CAD build for the part. Positions are in the model's coordinates, mm. A direction names the side the tool comes from. Coordinates: 2 decimals unless noted, no trailing zeros. Loops run counter-clockwise (first coordinate to the right, second up) from the corner with the lowest first, then second, coordinate; pieces in that order, holes last. Notation, with made-up numbers: (-31, -7.5) - (-11, -7.5) arc R19 cw to (-11, -1.5) - close; hole circle Ø2 at (26, -31.5). An arc over 180 degrees is marked (long way). Put each result on its own line as item: value.
```python
from build123d import *
from build123d.topology import SkipClean

# Parameters (mm, degrees)
SKETCH1_R           = 254.5
SKETCH1_R_2         = 234.5
BOSS_EXTRUDE1_DEPTH = 5
BOSS_EXTRUDE2_DEPTH = 500
SKETCH3_W           = 27.805822748
SKETCH3_H           = 60
CUT_EXTRUDE1_DEPTH  = 500
SKETCH4_R           = 250.5
CUT_EXTRUDE2_DEPTH  = 500
BOSS_EXTRUDE3_DEPTH = 500
BOSS_EXTRUDE4_DEPTH = 5
SKETCH11_W          = 21.416490723
SKETCH11_H          = 190
CUT_EXTRUDE3_DEPTH  = 10
CUT_EXTRUDE4_DEPTH  = 10
FILLET1_R           = 5
SKETCH15_R          = 2.5
CUT_EXTRUDE5_DEPTH  = 10
BOSS_EXTRUDE5_DEPTH = 3
SKETCH18_R          = 2.5
CUT_EXTRUDE6_DEPTH  = 5
CUT_EXTRUDE7_DEPTH  = 7
FILLET2_R           = 5
SKETCH21_R          = 2.5
CUT_EXTRUDE8_DEPTH  = 10
SKETCH22_R          = 2.5
CUT_EXTRUDE9_DEPTH  = 14
SKETCH23_R          = 5
CUT_EXTRUDE10_DEPTH = 3
SKETCH24_W          = 28.197779234
SKETCH24_H          = 25
CUT_EXTRUDE11_DEPTH = 45
FILLET3_R           = 2


with BuildPart() as part:
    # Sketch1 → Boss-Extrude1 (new body)
    with BuildSketch(Plane(origin=(0, 0, 0), x_dir=(1, 0, 0), z_dir=(0, 1, 0))):
        with Locations(Location((0, 0, 0), (0, 0, 270))):
            Circle(SKETCH1_R)
        with Locations(Location((0, 0, 0), (0, 0, 270))):
            Circle(SKETCH1_R_2, mode=Mode.SUBTRACT)
    extrude(amount=BOSS_EXTRUDE1_DEPTH)

    # Sketch2 → Boss-Extrude2 (add)
    with SkipClean():  # the faces are left unmerged after this step: merging them gives an invalid solid
        with BuildSketch(Plane(origin=(0, 5, 0), x_dir=(1, 0, 0), z_dir=(0, 1, 0))):
            with BuildLine():
                Line((254.5, 0), (234.5, 0))
                ThreePointArc((234.5, 0), (225.296071541, 65.053286992), (198.406779118, 125))
                Line((198.406779118, 125), (221.687279743, 125))
                ThreePointArc((221.687279743, 125), (246.16017417, 64.617479467), (254.5, 0))
            make_face()
        boss_extrude2 = extrude(amount=BOSS_EXTRUDE2_DEPTH)

    # Mirror1: Boss-Extrude2 across plane
    with SkipClean():  # the faces are left unmerged after this step: merging them gives an invalid solid
        add(boss_extrude2.mirror(Plane(origin=(0, 505, 0), x_dir=(1, 0, 0), z_dir=(0, 0, 1))))

    # Sketch3 → Cut-Extrude1 (cut)
    with SkipClean():  # the faces are left unmerged after this step: merging them gives an invalid solid
        with BuildSketch(Plane(origin=(0, 5, 0), x_dir=(1, 0, 0), z_dir=(0, 1, 0))):
            with Locations((-240.597088626, 30)):
                Rectangle(SKETCH3_W, SKETCH3_H)
        cut_extrude1 = extrude(amount=-CUT_EXTRUDE1_DEPTH, mode=Mode.SUBTRACT)

    # Mirror2: Cut-Extrude1 across plane
    with SkipClean():  # the faces are left unmerged after this step: merging them gives an invalid solid
        add(cut_extrude1.mirror(Plane.XY), mode=Mode.SUBTRACT)

    # Sketch4 → Cut-Extrude2 (cut)
    with SkipClean():  # the faces are left unmerged after this step: merging them gives an invalid solid
        with BuildSketch(Plane(origin=(0, 505, 0), x_dir=(1, 0, 0), z_dir=(0, 1, 0))):
            Circle(SKETCH4_R)
        extrude(amount=-CUT_EXTRUDE2_DEPTH, mode=Mode.SUBTRACT)

    # Sketch8 → Boss-Extrude3 (add)
    with SkipClean():  # the faces are left unmerged after this step: merging them gives an invalid solid
        with BuildSketch(Plane(origin=(0, 5, 0), x_dir=(1, 0, 0), z_dir=(0, 1, 0))):
            Polygon((217.083509277, 125), (168.583509277, 125), (168.583509277, 120), (220.045796136, 120), (220.045796136, 125), align=None)
        boss_extrude3 = extrude(amount=BOSS_EXTRUDE3_DEPTH)

    # Mirror3: Boss-Extrude3 across plane
    with SkipClean():  # the faces are left unmerged after this step: merging them gives an invalid solid
        add(boss_extrude3.mirror(Plane.XY))

    # Sketch10 → Boss-Extrude4 (add)
    with SkipClean():  # the faces are left unmerged after this step: merging them gives an invalid solid
        with BuildSketch(Plane.XZ):
            with BuildLine():
                Line((198.406779118, 125), (168.583509277, 125))
                Line((168.583509277, 125), (168.583509277, -125))
                Line((168.583509277, -125), (198.406779118, -125))
                ThreePointArc((198.406779118, -125), (234.5, 0), (198.406779118, 125))
            make_face()
        extrude(amount=-BOSS_EXTRUDE4_DEPTH)

    # Sketch11 → Cut-Extrude3 (cut)
    with SkipClean():  # the faces are left unmerged after this step: merging them gives an invalid solid
        with BuildSketch(Plane(origin=(0, 5, 0), x_dir=(1, 0, 0), z_dir=(0, 1, 0))):
            with Locations((179.291754639, -1.5)):
                Rectangle(SKETCH11_W, SKETCH11_H)
        extrude(amount=-CUT_EXTRUDE3_DEPTH, mode=Mode.SUBTRACT)

    # Sketch12 → Cut-Extrude4 (cut)
    with SkipClean():  # the faces are left unmerged after this step: merging them gives an invalid solid
        with BuildSketch(Plane(origin=(0, 5, 0), x_dir=(1, 0, 0), z_dir=(0, 1, 0))):
            with BuildLine():
                Line((213, 93.5), (190, 93.5))
                Line((190, 93.5), (190, 75))
                Line((190, 75), (213, 75))
                ThreePointArc((213, 75), (216.535533906, 76.464466094), (218, 80))
                Line((218, 80), (218, 88.5))
                ThreePointArc((218, 88.5), (216.535533906, 92.035533906), (213, 93.5))
            make_face()
            with BuildLine():
                Line((185, 120), (168.583509277, 120))
                Line((168.583509277, 120), (168.583509277, 93.5))
                Line((168.583509277, 93.5), (190, 93.5))
                Line((190, 93.5), (190, 115))
                ThreePointArc((190, 115), (188.535533906, 118.535533906), (185, 120))
            make_face()
            with BuildLine():
                ThreePointArc((213, -93.5), (216.535533906, -92.035533906), (218, -88.5))
                Line((218, -88.5), (218, -80))
                ThreePointArc((218, -80), (216.535533906, -76.464466094), (213, -75))
                Line((213, -75), (190, -75))
                Line((190, -75), (190, -93.5))
                Line((190, -93.5), (213, -93.5))
            make_face()
            with BuildLine():
                Line((190, -115), (190, -93.5))
                Line((190, -93.5), (168.583509277, -93.5))
                Line((168.583509277, -93.5), (168.583509277, -120))
                Line((168.583509277, -120), (185, -120))
                ThreePointArc((185, -120), (188.535533906, -118.535533906), (190, -115))
            make_face()
        extrude(amount=-CUT_EXTRUDE4_DEPTH, mode=Mode.SUBTRACT)

    # Fillet1
    fillet1_edges = [part.edges().sort_by_distance(p)[0] for p in [
        (190, 2.5, 75),
        (190, 2.5, 93.5),
        (190, 2.5, -93.5),
        (190, 2.5, -75),
    ]]
    fillet(fillet1_edges, radius=FILLET1_R)

    # Sketch15 → Cut-Extrude5 (cut)
    with BuildSketch(Plane(origin=(0, 5, 0), x_dir=(1, 0, 0), z_dir=(0, 1, 0))):
        with Locations(Location((242.5, 0, 0), (0, 0, 270))):
            Circle(SKETCH15_R)
        with Locations(Location((196.186621136, -142.537923681, 0), (0, 0, 270))):
            Circle(SKETCH15_R)
        with Locations(Location((74.936621136, -230.631205202, 0), (0, 0, 270))):
            Circle(SKETCH15_R)
        with Locations(Location((-74.936621136, -230.631205202, 0), (0, 0, 270))):
            Circle(SKETCH15_R)
        with Locations(Location((-196.186621136, -142.537923681, 0), (0, 0, 270))):
            Circle(SKETCH15_R)
        with Locations((-242.5, 0)):
            Circle(SKETCH15_R)
        with Locations(Location((-196.186621136, 142.537923681, 0), (0, 0, 270))):
            Circle(SKETCH15_R)
        with Locations(Location((-74.936621136, 230.631205202, 0), (0, 0, 270))):
            Circle(SKETCH15_R)
        with Locations(Location((74.936621136, 230.631205202, 0), (0, 0, 270))):
            Circle(SKETCH15_R)
        with Locations(Location((196.186621136, 142.537923681, 0), (0, 0, 270))):
            Circle(SKETCH15_R)
    extrude(amount=-CUT_EXTRUDE5_DEPTH, mode=Mode.SUBTRACT)

    # Sketch16 → Boss-Extrude5 (add)
    with SkipClean():  # the faces are left unmerged after this step: merging them gives an invalid solid
        with BuildSketch(Plane(origin=(0, 5, 0), x_dir=(1, 0, 0), z_dir=(0, 1, 0))):
            with BuildLine():
                Line((-247.326201604, 60), (-244.238101041, 60))
                ThreePointArc((-244.238101041, 60), (-35.003834494, 249.052166364), (218.236683443, 125))
                Line((218.236683443, 125), (221.687279743, 125))
                ThreePointArc((221.687279743, 125), (-34.936922855, 252.090581779), (-247.326201604, 60))
            make_face()
            with BuildLine():
                Line((221.687279743, -125), (218.236683443, -125))
                ThreePointArc((218.236683443, -125), (-35.003834494, -249.052166364), (-244.238101041, -60))
                Line((-244.238101041, -60), (-247.326201604, -60))
                ThreePointArc((-247.326201604, -60), (-34.936922855, -252.090581779), (221.687279743, -125))
            make_face()
        extrude(amount=BOSS_EXTRUDE5_DEPTH)

    # Sketch18 → Cut-Extrude6 (cut)
    with BuildSketch(Plane(origin=(0, 5, 0), x_dir=(1, 0, 0), z_dir=(0, 1, 0))):
        with Locations(Location((0, -242.5, 0), (0, 0, 270))):
            Circle(SKETCH18_R)
        with Locations(Location((-142.537923681, -196.186621136, 0), (0, 0, 270))):
            Circle(SKETCH18_R)
        with Locations(Location((-230.631205202, -74.936621136, 0), (0, 0, 270))):
            Circle(SKETCH18_R)
        with Locations(Location((-230.631205202, 74.936621136, 0), (0, 0, 270))):
            Circle(SKETCH18_R)
        with Locations(Location((-142.537923681, 196.186621136, 0), (0, 0, 270))):
            Circle(SKETCH18_R)
        with Locations(Location((0, 242.5, 0), (0, 0, 270))):
            Circle(SKETCH18_R)
        with Locations(Location((142.537923681, 196.186621136, 0), (0, 0, 270))):
            Circle(SKETCH18_R)
        with Locations(Location((230.631205202, 74.936621136, 0), (0, 0, 270))):
            Circle(SKETCH18_R)
        with Locations(Location((230.631205202, -74.936621136, 0), (0, 0, 270))):
            Circle(SKETCH18_R)
        with Locations(Location((142.537923681, -196.186621136, 0), (0, 0, 270))):
            Circle(SKETCH18_R)
    extrude(amount=-CUT_EXTRUDE6_DEPTH, mode=Mode.SUBTRACT)

    # Sketch19 → Cut-Extrude7 (cut)
    with BuildSketch(Plane.XZ):
        with BuildLine():
            Line((193, 20), (207, 20))
            ThreePointArc((207, 20), (209.121320344, 19.121320344), (210, 17))
            Line((210, 17), (210, -17))
            ThreePointArc((210, -17), (209.121320344, -19.121320344), (207, -20))
            Line((207, -20), (193, -20))
            Line((193, -20), (190, -20))
            Line((190, -20), (190, -17))
            Line((190, -17), (190, 17))
            Line((190, 17), (190, 20))
            Line((190, 20), (193, 20))
        make_face()
    extrude(amount=-CUT_EXTRUDE7_DEPTH, mode=Mode.SUBTRACT)

    # Fillet2
    fillet2_edges = [part.edges().sort_by_distance(p)[0] for p in [
        (190, 2.5, -20),
        (190, 2.5, 20),
    ]]
    fillet(fillet2_edges, radius=FILLET2_R)

    # Sketch21 → Cut-Extrude8 (cut)
    with SkipClean():  # the faces are left unmerged after this step: merging them gives an invalid solid
        with BuildSketch(Plane(origin=(0, 5, 0), x_dir=(1, 0, 0), z_dir=(0, 1, 0))):
            with Locations(Location((200, 50, 0), (0, 0, 270))):
                Circle(SKETCH21_R)
            with Locations(Location((200, -50, 0), (0, 0, 270))):
                Circle(SKETCH21_R)
        extrude(amount=-CUT_EXTRUDE8_DEPTH, mode=Mode.SUBTRACT)

    # Sketch22 → Cut-Extrude9 (cut)
    with SkipClean():  # the faces are left unmerged after this step: merging them gives an invalid solid
        with BuildSketch(Plane.XY.offset(125)):
            with Locations((181.083509277, 490)):
                Circle(SKETCH22_R)
            with Locations((181.083509277, 290)):
                Circle(SKETCH22_R)
            with Locations((181.083509277, 90)):
                Circle(SKETCH22_R)
        cut_extrude9 = extrude(amount=-CUT_EXTRUDE9_DEPTH, mode=Mode.SUBTRACT)

    # Mirror4: Cut-Extrude9 across plane
    with SkipClean():  # the faces are left unmerged after this step: merging them gives an invalid solid
        add(cut_extrude9.mirror(Plane.XY), mode=Mode.SUBTRACT)

    # Sketch23 → Cut-Extrude10 (cut)
    with SkipClean():  # the faces are left unmerged after this step: merging them gives an invalid solid
        with BuildSketch(Plane.XY.offset(125)):
            with Locations((181.083509277, 490)):
                Circle(SKETCH23_R)
            with Locations((181.083509277, 290)):
                Circle(SKETCH23_R)
            with Locations((181.083509277, 90)):
                Circle(SKETCH23_R)
        cut_extrude10 = extrude(amount=-CUT_EXTRUDE10_DEPTH, mode=Mode.SUBTRACT)

    # Mirror5: Cut-Extrude10 across plane
    with SkipClean():  # the faces are left unmerged after this step: merging them gives an invalid solid
        add(cut_extrude10.mirror(Plane.XY), mode=Mode.SUBTRACT)

    # Sketch24 → Cut-Extrude11 (cut, symmetric)
    with SkipClean():  # the faces are left unmerged after this step: merging them gives an invalid solid
        with BuildSketch(Plane.XY):
            with Locations((254.5, 246.5)):
                Rectangle(SKETCH24_W, SKETCH24_H)
        extrude(amount=CUT_EXTRUDE11_DEPTH, both=True, mode=Mode.SUBTRACT)

    # Fillet3
    fillet3_edges = [part.edges().sort_by_distance(p)[0] for p in [
        (248.457478811, 259, -45),
        (248.457478811, 234, -45),
        (248.457478811, 259, 45),
        (248.457478811, 234, 45),
    ]]
    fillet(fillet3_edges, radius=FILLET3_R)


solid = part.part
```
Q1. Pin check, flat tips, straight feed: pin 1 Ø1 at (y, z) = (75.5, 74.5) entering from -X; pin 2 Ø9 at (x, y) = (181.08, 290) entering from +Z; pin 3 Ø2.5 at (x, y) = (202.5, 2.5) entering from +Z. Stop position of each tip, or through.
Determined:
pin 1: x = 239.01
pin 2: z = 122
pin 3: z = 155.78
Q2. Slice it at C-C, the plane y = 160.5. Give the cut face in (x, z).
Determined:
outline: (168.58, -125) - (221.69, -125) arc R254.5 ccw to (221.69, 125) - (168.58, 125) - (168.58, 120) - (219.89, 120) arc R250.5 cw to (219.89, -120) - (168.58, -120) - close
Q3. Slice it at B-B, the plane z = -209. Give the cut face in (x, y), then the cut area to 3 significant figures.
Determined:
outline: (-145.22, 0) - (-106.34, 0) - (-106.34, 5) - (-139.9, 5) - (-139.9, 8) - (-145.22, 8) - close; (106.34, 0) - (145.22, 0) - (145.22, 8) - (139.9, 8) - (139.9, 5) - (106.34, 5) - close
area: 421 mm2
Q4. Wall check: L1, parallel to Z at x = 199.5, y = 452; L2, parallel to Z at x = 200, y = 3; L3, parallel to X at y = 490, z = -120.55. Give the ranges that are in metal, low to high. Write a range as from..to.
Determined:
L1: -125..-120, 120..125
L2: -157.39..-93.5, -75..-52.5, -47.5..-20, 20..47.5, 52.5..75, 93.5..157.39
L3: 168.58..178.58, 183.58..224.14
Q5. Slice it at A-A, the plane x = 22. Give the cut face in (y, z), then the cut area to 3 significant figures.
Determined:
outline: (0, -253.55) - (8, -253.55) - (8, -250.54) - (5, -250.54) - (5, -233.47) - (0, -233.47) - close; (0, 233.47) - (5, 233.47) - (5, 250.54) - (8, 250.54) - (8, 253.55) - (0, 253.55) - close
area: 219 mm2
Q6. Mould opens along X. For faces 1 (the cylindrical face through (-31.67, 2.46, -232.35)), 2 (the flat face through (207, 0, 39)) say: +X half, -X half, draft (parallel to the pull), parting line (faces both ways), or undercut.
Determined:
face 1: undercut
face 2: draft
Q7. Tool access for faces 3 (the flat face through (250, 505, 38)), 4 (the cylindrical face through (-39.149, 6.479, -248.434)): list every direction of +Z, -Z, +X, -X, +Y, -Y with a clear straight run to the whole face (end or side of a thin tool).
Determined:
face 3: +Z, -Z, +X, -X, +Y
face 4: +Y
